CAD build for the part. Positions are in the model's coordinates, mm. Face numbers are marked on the shaded views. A direction names the side the tool comes from. Round coordinates to 2 decimals unless told otherwise and drop trailing zeros. Loops run counter-clockwise (first coordinate to the right, second up) from the corner with the lowest first, then second, coordinate; pieces in that order, holes last.
```python
from build123d import *

# Parameters (mm, degrees)
SKETCH1_R           = 65
SKETCH1_R_2         = 55
BOSS_EXTRUDE1_DEPTH = 100
BOSS_EXTRUDE2_START = 20
SKETCH3_R           = 55
SKETCH3_R_2         = 20
SKETCH3_R_3         = 13
BOSS_EXTRUDE2_DEPTH = 20
BOSS_EXTRUDE3_START = 60
SKETCH3_5_R         = 55
SKETCH3_5_R_2       = 20
SKETCH3_5_R_3       = 13
SKETCH3_5_R_4       = 6.5
BOSS_EXTRUDE3_DEPTH = 20
BOSS_EXTRUDE4_START = 20
SKETCH3_7_R         = 13
BOSS_EXTRUDE4_DEPTH = 60
SKETCH3_10_R        = 13
BOSS_EXTRUDE5_DEPTH = 20
BOSS_EXTRUDE6_START = 80
SKETCH3_11_R        = 13
BOSS_EXTRUDE6_DEPTH = 20


with BuildPart() as part:
    # Sketch1 → Boss-Extrude1 (new body)
    with BuildSketch(Plane(origin=(0, 0, 0), x_dir=(1, 0, 0), z_dir=(0, 1, 0))):
        with Locations(Location((0, 0, 0), (0, 0, 270))):
            Circle(SKETCH1_R)
        with Locations(Location((0, 0, 0), (0, 0, 270))):
            Circle(SKETCH1_R_2, mode=Mode.SUBTRACT)
    extrude(amount=BOSS_EXTRUDE1_DEPTH)

    # Sketch3 → Boss-Extrude2 (add)
    with BuildSketch(Plane(origin=(0, 0, 0), x_dir=(1, 0, 0), z_dir=(0, 1, 0)).offset(BOSS_EXTRUDE2_START)):
        with Locations(Location((0, 0, 0), (0, 0, 270))):
            Circle(SKETCH3_R)
        with BuildLine():
            ThreePointArc((39.298819185, 16.181866723), (42.375869887, 3.245866806), (41.304875194, -10.00786117))
            Line((41.304875194, -10.00786117), (19.437588327, -4.709581727))
            ThreePointArc((19.437588327, -4.709581727), (17.030904249, -10.485623513), (12.957116602, -15.235259412))
            Line((12.957116602, -15.235259412), (27.53387278, -32.374926251))
            ThreePointArc((27.53387278, -32.374926251), (16.181866723, -39.298819185), (3.245866806, -42.375869887))
            Line((3.245866806, -42.375869887), (1.527466732, -19.941585829))
            ThreePointArc((1.527466732, -19.941585829), (-4.709581727, -19.437588327), (-10.485623513, -17.030904249))
            Line((-10.485623513, -17.030904249), (-22.281949965, -36.190671529))
            ThreePointArc((-22.281949965, -36.190671529), (-32.374926251, -27.53387278), (-39.298819185, -16.181866723))
            Line((-39.298819185, -16.181866723), (-18.493561969, -7.614996105))
            ThreePointArc((-18.493561969, -7.614996105), (-19.941585829, -1.527466732), (-19.437588327, 4.709581727))
            Line((-19.437588327, 4.709581727), (-41.304875194, 10.00786117))
            ThreePointArc((-41.304875194, 10.00786117), (-36.190671529, 22.281949965), (-27.53387278, 32.374926251))
            Line((-27.53387278, 32.374926251), (-12.957116602, 15.235259412))
            ThreePointArc((-12.957116602, 15.235259412), (-7.614996105, 18.493561969), (-1.527466732, 19.941585829))
            Line((-1.527466732, 19.941585829), (-3.245866806, 42.375869887))
            ThreePointArc((-3.245866806, 42.375869887), (10.00786117, 41.304875194), (22.281949965, 36.190671529))
            Line((22.281949965, 36.190671529), (10.485623513, 17.030904249))
            ThreePointArc((10.485623513, 17.030904249), (15.235259412, 12.957116602), (18.493561969, 7.614996105))
            Line((18.493561969, 7.614996105), (39.298819185, 16.181866723))
        make_face(mode=Mode.SUBTRACT)
        Circle(SKETCH3_R_2)
        with Locations(Location((0, 0, 0), (0, 0, 270))):
            Circle(SKETCH3_R_3, mode=Mode.SUBTRACT)
    extrude(amount=BOSS_EXTRUDE2_DEPTH)

    # Sketch3_5 → Boss-Extrude3 (add)
    with BuildSketch(Plane(origin=(0, 0, 0), x_dir=(1, 0, 0), z_dir=(0, 1, 0)).offset(BOSS_EXTRUDE3_START)):
        with Locations(Location((0, 0, 0), (0, 0, 270))):
            Circle(SKETCH3_5_R)
        with BuildLine():
            ThreePointArc((39.298819185, 16.181866723), (42.375869887, 3.245866806), (41.304875194, -10.00786117))
            Line((41.304875194, -10.00786117), (19.437588327, -4.709581727))
            ThreePointArc((19.437588327, -4.709581727), (17.030904249, -10.485623513), (12.957116602, -15.235259412))
            Line((12.957116602, -15.235259412), (27.53387278, -32.374926251))
            ThreePointArc((27.53387278, -32.374926251), (16.181866723, -39.298819185), (3.245866806, -42.375869887))
            Line((3.245866806, -42.375869887), (1.527466732, -19.941585829))
            ThreePointArc((1.527466732, -19.941585829), (-4.709581727, -19.437588327), (-10.485623513, -17.030904249))
            Line((-10.485623513, -17.030904249), (-22.281949965, -36.190671529))
            ThreePointArc((-22.281949965, -36.190671529), (-32.374926251, -27.53387278), (-39.298819185, -16.181866723))
            Line((-39.298819185, -16.181866723), (-18.493561969, -7.614996105))
            ThreePointArc((-18.493561969, -7.614996105), (-19.941585829, -1.527466732), (-19.437588327, 4.709581727))
            Line((-19.437588327, 4.709581727), (-41.304875194, 10.00786117))
            ThreePointArc((-41.304875194, 10.00786117), (-36.190671529, 22.281949965), (-27.53387278, 32.374926251))
            Line((-27.53387278, 32.374926251), (-12.957116602, 15.235259412))
            ThreePointArc((-12.957116602, 15.235259412), (-7.614996105, 18.493561969), (-1.527466732, 19.941585829))
            Line((-1.527466732, 19.941585829), (-3.245866806, 42.375869887))
            ThreePointArc((-3.245866806, 42.375869887), (10.00786117, 41.304875194), (22.281949965, 36.190671529))
            Line((22.281949965, 36.190671529), (10.485623513, 17.030904249))
            ThreePointArc((10.485623513, 17.030904249), (15.235259412, 12.957116602), (18.493561969, 7.614996105))
            Line((18.493561969, 7.614996105), (39.298819185, 16.181866723))
        make_face(mode=Mode.SUBTRACT)
        Circle(SKETCH3_5_R_2)
        with Locations(Location((0, 0, 0), (0, 0, 270))):
            Circle(SKETCH3_5_R_3, mode=Mode.SUBTRACT)
        Circle(SKETCH3_5_R_4)
    extrude(amount=BOSS_EXTRUDE3_DEPTH)


with BuildPart() as boss_extrude3_kept_piece:
    # of the separate pieces the step leaves, the one the design keeps (boss_extrude3_pieces_kept)
    add(part.part.solids().sort_by_distance((0, 0, 65))[0])

    # Sketch3_7 → Boss-Extrude4 (add)
    with BuildSketch(Plane(origin=(0, 0, 0), x_dir=(1, 0, 0), z_dir=(0, 1, 0)).offset(BOSS_EXTRUDE4_START)):
        with Locations(Location((0, 0, 0), (0, 0, 270))):
            Circle(SKETCH3_7_R)
        with BuildLine():
            Line((2, 8.5), (2, 6.184658438))
            ThreePointArc((2, 6.184658438), (5.25594901, 3.824264635), (6.5, 0))
            ThreePointArc((6.5, 0), (-3.824264635, -5.25594901), (-2, 6.184658438))
            Line((-2, 6.184658438), (-2, 8.5))
            Line((-2, 8.5), (2, 8.5))
        make_face(mode=Mode.SUBTRACT)
        with BuildLine():
            ThreePointArc((-2, 6.184658438), (0, 6.5), (2, 6.184658438))
            Line((2, 6.184658438), (2, 8.5))
            Line((2, 8.5), (-2, 8.5))
            Line((-2, 8.5), (-2, 6.184658438))
        make_face()
    extrude(amount=BOSS_EXTRUDE4_DEPTH)

    # Sketch3_10 → Boss-Extrude5 (add)
    with BuildSketch(Plane(origin=(0, 0, 0), x_dir=(1, 0, 0), z_dir=(0, 1, 0))):
        with Locations(Location((0, 0, 0), (0, 0, 270))):
            Circle(SKETCH3_10_R)
        with BuildLine():
            Line((2, 5.656854249), (2, 8.5))
            Line((2, 8.5), (-2, 8.5))
            Line((-2, 8.5), (-2, 5.656854249))
            ThreePointArc((-2, 5.656854249), (0, -6), (2, 5.656854249))
        make_face(mode=Mode.SUBTRACT)
    extrude(amount=BOSS_EXTRUDE5_DEPTH)

    # Sketch3_11 → Boss-Extrude6 (add)
    with BuildSketch(Plane(origin=(0, 0, 0), x_dir=(1, 0, 0), z_dir=(0, 1, 0)).offset(BOSS_EXTRUDE6_START)):
        with Locations(Location((0, 0, 0), (0, 0, 270))):
            Circle(SKETCH3_11_R)
        with BuildLine():
            Line((2, 5.656854249), (2, 8.5))
            Line((2, 8.5), (-2, 8.5))
            Line((-2, 8.5), (-2, 5.656854249))
            ThreePointArc((-2, 5.656854249), (0, -6), (2, 5.656854249))
        make_face(mode=Mode.SUBTRACT)
    extrude(amount=BOSS_EXTRUDE6_DEPTH)


solid = boss_extrude3_kept_piece.part
```
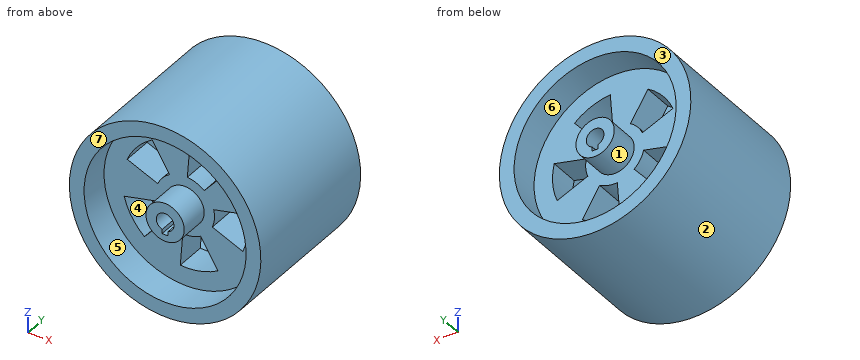
Item 1: Cut at A-A, the plane y = 16. Give the cut face in (x, z).
Answers follow:
outline: circle Ø130 at (0, 0); circle Ø26 at (0, 0); hole circle Ø110 at (0, 0); hole (-2, -8.5) - (2, -8.5) - (2, -5.66) arc R6 ccw (long way) to (-2, -5.66) - close
Item 2: Two-plate mould, pull along Z, no slides. Class the marked faces 1, 2 and 3: released by +Z, released by -Z, zero draft, split by the parting line, or undercut.
Answers follow:
face 1: undercut
face 2: split by the parting line
face 3: zero draft
Item 3: Probe line 1 (X direction, y = 86.5, z = 0); line 2 (Y direction, x = 44, z = -11.5); line 3 (Z direction, x = -26, y = 67). List the from-to ranges inside material, lowest first.
Answers follow:
line 1: x = -65 to -55, -13 to -6, 6 to 13, 55 to 65
line 2: y = 20 to 40, 60 to 80
line 3: z = -59.57 to -30.57, -6.3 to 10.71, 33.62 to 59.57
Item 4: Flat gauge pins, fed straight in: P1, Ø3, axis at y = 87.5, z = 48.5, coming from the -X side; P2, Ø3, axis at y = 70.5, z = 39, coming from the -X side; P3, Ø5, axis at x = 32.5, y = 67, coming from the -Z side. Where does each tip first touch, or does it go through?
Answers follow:
P1: stops at x = -44.9
P2: stops at x = -53.09
P3: stops at z = -57.66
Item 5: Cut at B-B, the plane x = -33.5. State how many separate pieces and enclosed holes the cut face has, plus the area to 3 significant figures.
Answers follow:
separate pieces: 4
enclosed holes: 0
area: 4,690 mm2
Item 6: Cut at C-C, the plane y = 49.5. Give the cut face in (x, z), plus the area to 3 significant figures.
Answers follow:
outline: circle Ø130 at (0, 0); circle Ø26 at (0, 0); hole circle Ø110 at (0, 0); hole circle Ø13 at (0, 0)
area: 4,170 mm2
Item 7: 3-axis set-ups, long thin cutter, end or side, ignore diameter. For the marked faces 4, 5, 6 and 7: which of +Z, -Z, +X, -X, +Y, -Y reach the whole face in a straight line?
Answers follow:
face 4: +Y, -Y
face 5: -Y
face 6: +Y
face 7: +Z, -Z, +X, -X, -Y
Item 8: Cut at D-D, the plane y = 70. Give the cut face in (x, z) (3 decimals), plus the area to 3 significant figures.
Answers follow:
outline: circle Ø130 at (0, 0); hole (-41.305, -10.008) arc R42.5 ccw to (-27.534, -32.375) - (-12.957, -15.235) arc R20 cw to (-19.438, -4.71) - close; hole (-39.299, 16.182) - (-18.494, 7.615) arc R20 cw to (-10.486, 17.031) - (-22.282, 36.191) arc R42.5 ccw to start; hole circle Ø13 at (0, 0); hole (-3.246, -42.376) arc R42.5 ccw to (22.282, -36.191) - (10.486, -17.031) arc R20 cw to (-1.527, -19.942) - close; hole (1.527, 19.942) arc R20 cw to (12.957, 15.235) - (27.534, 32.375) arc R42.5 ccw to (3.246, 42.376) - close; hole (18.494, -7.615) - (39.299, -16.182) arc R42.5 ccw to (41.305, 10.008) - (19.438, 4.71) arc R20 cw to start
area: 10,900 mm2
